Could you check a few things on this model? Use its own coordinates, in mm. Face numbers are marked on the shaded views. A direction names the side the tool comes from. Give positions to 0.01 mm unless a question says otherwise; leave off trailing zeros. Order: outer loops, then holes, each group sorted by start corner. A loop starts at its lowest first (then second) coordinate and runs counter-clockwise, first axis right, second up. Notation, with made-up numbers: (-0.5, 86.25) -> (5.5, 86.25) arc R21 cw to (5.5, 119.25) -> close; hole circle Ø10 at (39, 37). An arc over 180 degrees is marked (long way). Use one line per item in the form item = value. Start each with the question number.
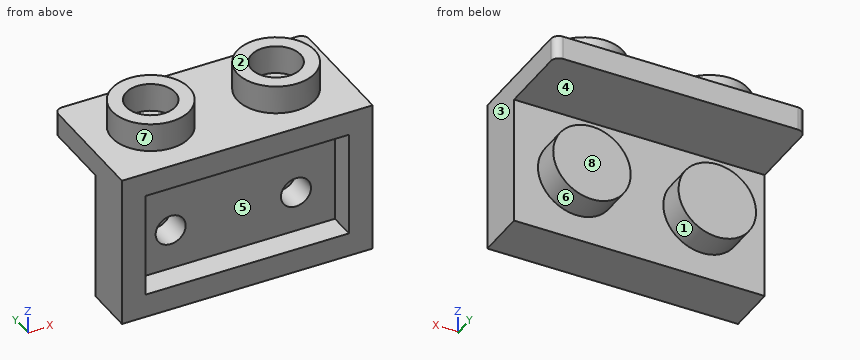
from build123d import *

# Parameters (mm, degrees)
BOSS_EXTRUDE1_DEPTH = 15.85
SKETCH2_R           = 2.45
SKETCH2_R_2         = 1.55
BOSS_EXTRUDE2_DEPTH = 1.8
SKETCH3_R           = 2.45
BOSS_EXTRUDE3_DEPTH = 1.8
SHELL1_OUTLINE_W    = 12.85
SHELL1_OUTLINE_H    = 6.65
SHELL1_DEPTH        = 1.65
SHELL1_START        = 1.65
SHELL1_2_OUTLINE_R  = 0.95
SHELL1_2_DEPTH      = 1.8
FILLET1_R           = 0.5


# Read off the part's stored shape, not the designer's step: Shell1
with BuildPart() as part:
    # Sketch1 → Boss-Extrude1 (new body)
    with BuildSketch(Plane(origin=(0, 0, 0), x_dir=(0, 0, -1), z_dir=(1, 0, 0))):
        Polygon((0, 0), (0, 8), (1.5, 8), (1.5, 3.15), (9.65, 3.15), (9.65, 0), align=None)
    extrude(amount=-BOSS_EXTRUDE1_DEPTH)

    # Sketch2 → Boss-Extrude2 (add)
    # profile 1 of 2: a face of its own
    with BuildSketch(Plane.XY):
        with Locations((-11.8875, 4)):
            Circle(SKETCH2_R)
        with Locations((-11.8875, 4)):
            Circle(SKETCH2_R_2, mode=Mode.SUBTRACT)
    # profile 2 of 2: a face of its own
    with BuildSketch(Plane.XY):
        with Locations((-3.9625, 4)):
            Circle(SKETCH2_R)
        with Locations((-3.9625, 4)):
            Circle(SKETCH2_R_2, mode=Mode.SUBTRACT)
    extrude(amount=BOSS_EXTRUDE2_DEPTH)

    # Sketch3 → Boss-Extrude3 (add)
    with BuildSketch(Plane(origin=(0, 3.15, 0), x_dir=(1, 0, 0), z_dir=(0, 1, 0))):
        with Locations(Location((-11.8875, 5.575, 0), (0, 0, 270))):
            Circle(SKETCH3_R)
        with Locations(Location((-3.9625, 5.575, 0), (0, 0, 270))):
            Circle(SKETCH3_R)
    extrude(amount=BOSS_EXTRUDE3_DEPTH)

    # Shell1 outline → Shell1 (cut)
    with BuildSketch(Plane(origin=(0, 0, 0), x_dir=(1, 0, 0), z_dir=(0, 1, 0))):
        with Locations((-7.925, 4.825)):
            Rectangle(SHELL1_OUTLINE_W, SHELL1_OUTLINE_H)
    extrude(amount=SHELL1_DEPTH, mode=Mode.SUBTRACT)

    # Shell1 2 outline → Shell1 2 (cut)
    with BuildSketch(Plane(origin=(0, 0, 0), x_dir=(1, 0, 0), z_dir=(0, 1, 0)).offset(SHELL1_START)):
        with Locations((-11.8875, 5.575)):
            Circle(SHELL1_2_OUTLINE_R)
        with Locations((-3.9625, 5.575)):
            Circle(SHELL1_2_OUTLINE_R)
    extrude(amount=SHELL1_2_DEPTH, mode=Mode.SUBTRACT)

    # Fillet1
    fillet1_edges = [part.edges().sort_by_distance(p)[0] for p in [
        (-15.85, 8, -0.75),
        (0, 8, -0.75),
    ]]
    fillet(fillet1_edges, radius=FILLET1_R)


solid = part.part
(1) Imagine slicing it at D-D (y = 5.25). Write out the boundary of the cut face in (x, z).
(2) We'd pull the mould along X, two halves only. Please class the marked faces 1, 2 and 3: pulls with the +X half, pulls with the -X half, needs draft (parallel to the pull), parting line crosses it, or undercut.
(3) I'm going to push flat-ended pins straight in: pin 1 Ø3 at (x, z) = (-11.89, -5.58) entering from -Y; pin 2 Ø4 at (x, z) = (-12, -6.5) entering from +Y; pin 3 Ø3 at (x, y) = (-11.89, 4) entering from +Z. Where does each tip first touch, or does it pass through?
(4) Please list where these lines run through material, in increasing order: probe 1 along X at (y, z) = (3.25, -5.25); probe 2 along Z at (x, y) = (-7.5, 1.5); probe 3 along Z at (x, y) = (-12, 3.25).
(5) Imagine slicing it at C-C (z = -1.75). Write out the boundary of the cut face in (x, y), plus the area to 3 significant figures.
(6) Imagine slicing it at B-B (x = -7.5). Write out the boundary of the cut face in (y, z).
(7) Which directions (+Z, -Z, +X, -X, +Y, -Y) give clear straight access to the entire face, cutting with the end or side of a thin tool? Please do the marked faces 4, 5, 6, 7 and 8.
(8) Imagine slicing it at A-A (y = 4). Give the number of separate pieces and of enclosed holes in the cut face, plus the area to 3 significant figures.
Calculated:
q1.outline = (-15.85, -1.5) -> (0, -1.5) -> (0, 0) -> (-1.86, 0) -> (-1.86, 1.8) -> (-3.05, 1.8) -> (-3.05, 0) -> (-4.88, 0) -> (-4.88, 1.8) -> (-6.07, 1.8) -> (-6.07, 0) -> (-9.78, 0) -> (-9.78, 1.8) -> (-10.97, 1.8) -> (-10.97, 0) -> (-12.8, 0) -> (-12.8, 1.8) -> (-13.99, 1.8) -> (-13.99, 0) -> (-15.85, 0) -> close
q2.face_1 = undercut
q2.face_2 = needs draft
q2.face_3 = pulls with the +X half
q3.pin_1 = 1.65
q3.pin_2 = 4.95
q3.pin_3 = 0
q4.probe_1 = -14.32 to -12.78, -10.99 to -9.46, -6.39 to -4.86, -3.07 to -1.53
q4.probe_2 = -9.65 to -8.15, -1.5 to 0
q4.probe_3 = -8.02 to -6.52, -4.63 to -3.13, -1.5 to 0
q5.outline = (-15.85, 0) -> (-14.35, 0) -> (-14.35, 1.65) -> (-1.5, 1.65) -> (-1.5, 0) -> (0, 0) -> (0, 3.15) -> (-15.85, 3.15) -> close
q5.area = 28.7 mm2
q6.outline = (0, -9.65) -> (3.15, -9.65) -> (3.15, -1.5) -> (8, -1.5) -> (8, 0) -> (0, 0) -> (0, -1.5) -> (1.65, -1.5) -> (1.65, -8.15) -> (0, -8.15) -> close
q7.face_4 = +X, -X, +Y
q7.face_5 = -Y
q7.face_6 = +Y
q7.face_7 = +Z
q7.face_8 = -Z, +X, -X, +Y
q8.separate_pieces = 3
q8.enclosed_holes = 0
q8.area = 68.0 mm2
